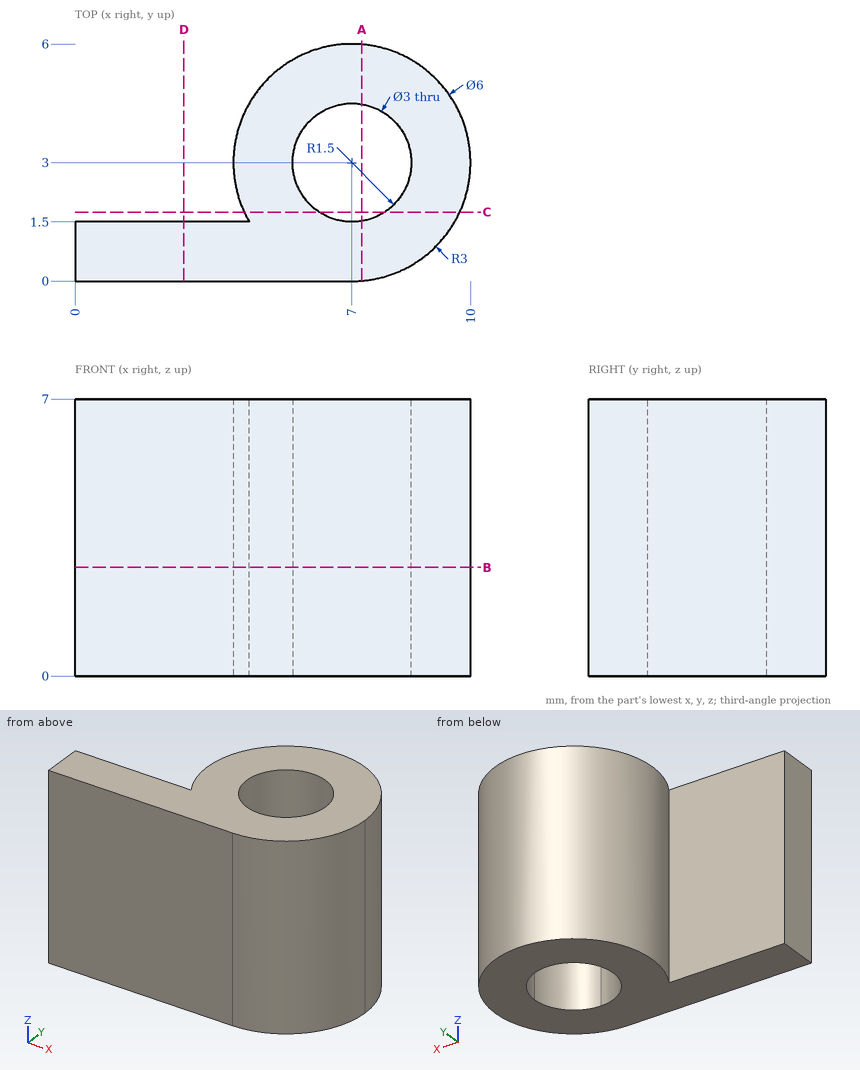
Source: three-view drawing plus pictorial views. Frame: mm from the lowest corner of the part. Give positions to 0.01 mm unless a question says otherwise; leave off trailing zeros. Loops run counter-clockwise (first coordinate to the right, second up) from the corner with the lowest first, then second, coordinate; pieces in that order, holes last. Notation, with made-up numbers: M -7.5,70 L 41.5,70 A10 ccw 41.5,81 Z; hole C 6,-0.5 d2. An arc over 180 degrees is marked long. Use CSV: the item, a comma, the result in double quotes.
(1) Section A-A, the plane x = 7.25. Return loops of the section in (y, z), plus the area to 3 significant figures.
Outcome:
outline,"M 0.01,0 L 1.52,0 L 1.52,7 L 0.01,7 Z; M 4.48,0 L 5.99,0 L 5.99,7 L 4.48,7 Z"
area,"21.1 mm²"
(2) Material intervals for L1, parallel to Y at x = 7, z = 4; L2, parallel to Y at x = 2, z = 1.5; L3, parallel to X at y = 2.5, z = 5.5, sorted ascending. Write a range as [from, to].
Outcome:
L1,"y = [0, 1.5], [4.5, 6]"
L2,"y = [0, 1.5]"
L3,"x = [4.04, 5.59], [8.41, 9.96]"
(3) Section D-D, the plane x = 2.75. Return loops of the section in (y, z).
Outcome:
outline,"M 0,0 L 1.5,0 L 1.5,7 L 0,7 Z"
(4) Section B-B, the plane z = 2.75. Return loops of the section in (x, y).
Outcome:
outline,"M 0,0 L 7,0 A3 ccw long 4.4,1.5 L 0,1.5 Z; hole C 7,3 d3"
(5) Section C-C, the plane y = 1.75. Return loops of the section in (x, z).
Outcome:
outline,"M 4.27,0 L 6.17,0 L 6.17,7 L 4.27,7 Z; M 7.83,0 L 9.73,0 L 9.73,7 L 7.83,7 Z"
(6) Pin query (flat end, axial travel): P1, Ø1.5, axis at y = 2.5, z = 2, coming from the -X side; P2, Ø1, axis at y = 1.5, z = 3.5, coming from the +X side; P3, Ø1, axis at x = 2, z = 1, coming from the +Y side. Return the tip coordinate at first contact, or that it passes through.
Outcome:
P1,"stops at x = 4"
P2,"stops at x = 9.83"
P3,"stops at y = 1.5"
